```python
from build123d import *

# Parameters (mm, degrees)
SKETCH1_W           = 350
SKETCH1_H           = 10
CHAMFER1_SIZE       = 0.5
SKETCH2_W           = 20
SKETCH2_H           = 6
BOSS_EXTRUDE1_DEPTH = 3.5
FILLET1_RADIUS      = 3
FILLET1_LENGTH      = 3.5
FILLET2_RADIUS      = 3
FILLET2_LENGTH      = 3.5
FILLET3_R           = 0.2
SKETCH4_W           = 20
SKETCH4_H           = 6
BOSS_EXTRUDE3_DEPTH = 3.5
FILLET4_RADIUS      = 3
FILLET4_LENGTH      = 3.5
FILLET5_RADIUS      = 3
FILLET5_LENGTH      = 3.5
FILLET6_R           = 0.2


with BuildPart() as part:
    # Sketch1 → Revolve1 (revolve)
    with BuildSketch(Plane.XY, mode=Mode.PRIVATE) as revolve1_sk:
        with Locations((175, 5)):
            Rectangle(SKETCH1_W, SKETCH1_H)
    revolve(revolve1_sk.sketch.rotate(Axis((0, 0, 0), (1, 0, 0)), 90), axis=Axis((0, 0, 0), (1, 0, 0)))

    # Chamfer1
    chamfer1_edges = [part.edges().sort_by_distance(p)[0] for p in [
        (0, 0, -10),
        (350, 0, -10),
    ]]
    chamfer(chamfer1_edges, length=CHAMFER1_SIZE)


with BuildPart() as body_2:
    # Sketch2 → Boss-Extrude1 (new body)
    with BuildSketch(Plane.XY.offset(10)):
        with Locations((160, 0)):
            Rectangle(SKETCH2_W, SKETCH2_H)
    extrude(amount=-BOSS_EXTRUDE1_DEPTH)

    # Fillet1: full round fillet: the end face becomes a half cylinder, R = half its width
    fillet1_face = Plane((150, 0, 8.25), x_dir=(0, 0, 1), z_dir=(-1, 0, 0))  # on the end face: x along it, z out of the body
    fillet1_slab = fillet1_face.offset(-FILLET1_RADIUS / 2) * Box(FILLET1_LENGTH, 2 * FILLET1_RADIUS, FILLET1_RADIUS, mode=Mode.PRIVATE)  # the body's end, R deep
    fillet1_round = Plane((153, 0, 8.25), x_dir=(-1, 0, 0), z_dir=(0, 0, 1)) * Cylinder(FILLET1_RADIUS, FILLET1_LENGTH, mode=Mode.PRIVATE)  # its axis R under the face
    add(fillet1_slab - fillet1_round, mode=Mode.SUBTRACT)

    # Fillet2: full round fillet: the end face becomes a half cylinder, R = half its width
    fillet2_face = Plane((170, 0, 8.25), x_dir=(0, 0, 1), z_dir=(1, 0, 0))  # on the end face: x along it, z out of the body
    fillet2_slab = fillet2_face.offset(-FILLET2_RADIUS / 2) * Box(FILLET2_LENGTH, 2 * FILLET2_RADIUS, FILLET2_RADIUS, mode=Mode.PRIVATE)  # the body's end, R deep
    fillet2_round = Plane((167, 0, 8.25), x_dir=(1, 0, 0), z_dir=(0, 0, 1)) * Cylinder(FILLET2_RADIUS, FILLET2_LENGTH, mode=Mode.PRIVATE)  # its axis R under the face
    add(fillet2_slab - fillet2_round, mode=Mode.SUBTRACT)

    # Fillet3
    fillet3_edges = [body_2.edges().sort_by_distance(p)[0] for p in [
        (160, -3, 6.5),
        (150, 0, 6.5),
        (160, 3, 6.5),
        (170, 0, 6.5),
    ]]
    fillet(fillet3_edges, radius=FILLET3_R)


with BuildPart() as part_1:
    add(part.part)

    # Combine1: cut body 2
    add(body_2.part, mode=Mode.SUBTRACT)


with BuildPart() as body_2_2:
    # Sketch4 → Boss-Extrude3 (new body)
    with BuildSketch(Plane.XY.offset(10)):
        with Locations((210, 0)):
            Rectangle(SKETCH4_W, SKETCH4_H)
    extrude(amount=-BOSS_EXTRUDE3_DEPTH)

    # Fillet4: full round fillet: the end face becomes a half cylinder, R = half its width
    fillet4_face = Plane((200, 0, 8.25), x_dir=(0, 0, 1), z_dir=(-1, 0, 0))  # on the end face: x along it, z out of the body
    fillet4_slab = fillet4_face.offset(-FILLET4_RADIUS / 2) * Box(FILLET4_LENGTH, 2 * FILLET4_RADIUS, FILLET4_RADIUS, mode=Mode.PRIVATE)  # the body's end, R deep
    fillet4_round = Plane((203, 0, 8.25), x_dir=(-1, 0, 0), z_dir=(0, 0, 1)) * Cylinder(FILLET4_RADIUS, FILLET4_LENGTH, mode=Mode.PRIVATE)  # its axis R under the face
    add(fillet4_slab - fillet4_round, mode=Mode.SUBTRACT)

    # Fillet5: full round fillet: the end face becomes a half cylinder, R = half its width
    fillet5_face = Plane((220, 0, 8.25), x_dir=(0, 0, -1), z_dir=(1, 0, 0))  # on the end face: x along it, z out of the body
    fillet5_slab = fillet5_face.offset(-FILLET5_RADIUS / 2) * Box(FILLET5_LENGTH, 2 * FILLET5_RADIUS, FILLET5_RADIUS, mode=Mode.PRIVATE)  # the body's end, R deep
    fillet5_round = Plane((217, 0, 8.25), x_dir=(1, 0, 0), z_dir=(0, 0, -1)) * Cylinder(FILLET5_RADIUS, FILLET5_LENGTH, mode=Mode.PRIVATE)  # its axis R under the face
    add(fillet5_slab - fillet5_round, mode=Mode.SUBTRACT)

    # Fillet6
    fillet6_edges = [body_2_2.edges().sort_by_distance(p)[0] for p in [
        (210, -3, 6.5),
        (200, 0, 6.5),
        (210, 3, 6.5),
        (220, 0, 6.5),
    ]]
    fillet(fillet6_edges, radius=FILLET6_R)


with BuildPart() as part_2:
    add(part_1.part)

    # Combine2: cut body 2 2
    add(body_2_2.part, mode=Mode.SUBTRACT)


solid = part_2.part
```
For this review, take the finished solid that the model builds, in its own axes (mm). A direction names the side the tool comes from. Round coordinates to 2 decimals unless told otherwise and drop trailing zeros. Write each loop counter-clockwise with the first axis right and the second up, starting at its lowest first coordinate (ties: lowest second). Pieces come first, ordered by that corner, then holes. Notation, with made-up numbers: (-33.5, 65) -> (-13.5, 65) arc R24 cw to (-13.5, 90) -> close; hole circle Ø4 at (58, 20.5). An arc over 180 degrees is marked (long way). One line per question, with ' | ' between items. Start each with the question number.
(1) Add section A-A, the plane x = 272.5. Write out the cut boundary in (y, z).
(2) Add section B-B, the plane x = 159. Write out the cut boundary in (y, z).
(3) Mouldability with a two-part tool opening along Y and no side actions: class faces 1 (the face through (160, 0, 6.5)), 2 (the face through (350, 0, 0)), 3 (the face through (177, 0, -10)) as released by +Y, released by -Y, zero draft, split by the parting line, or undercut.
(4) Tool access review of faces 4 (the face through (210, 0, 6.5)), 5 (the face through (0, 0, 0)): name each direction out of +Z, -Z, +X, -X, +Y, -Y from which nothing blocks a thin tool from reaching the whole face with its end or side.
(5) Insertion check: P1, Ø8, axis at x = 51.5, z = -7.5, coming from the -Y side; P2, Ø2.5, axis at x = 209.5, z = 8.5, coming from the +Y side; P3, Ø4.5, axis at x = 158, y = 0.5, coming from the +Z side. Each pin has a flat end and moves straight along its axis. Give the tip position at first contact, or say it passes through.
(6) For line 1 along Y through (x, z) = (166, 0); line 2 along Z through (x, y) = (71.5, 0.75); line 3 along Y through (x, z) = (222, 4.75), list the stretches that pass through material, from the lowest coordinate up. Write a range as from..to.
Answer list:
1) outline: circle Ø20 at (0, 0)
2) outline: (-3, 6.7) -> (-3, 9.54) arc R10 ccw (long way) to (3, 9.54) -> (3, 6.7) arc R0.2 cw to (2.8, 6.5) -> (-2.8, 6.5) arc R0.2 cw to start
3) face 1: undercut | face 2: zero draft | face 3: split by the parting line
4) face 4: +Z | face 5: +Z, -Z, -X, +Y, -Y
5) P1: y = -9.37 | P2: y = 6.89 | P3: z = 6.5
6) line 1: -10..10 | line 2: -9.97..9.97 | line 3: -8.8..8.8
